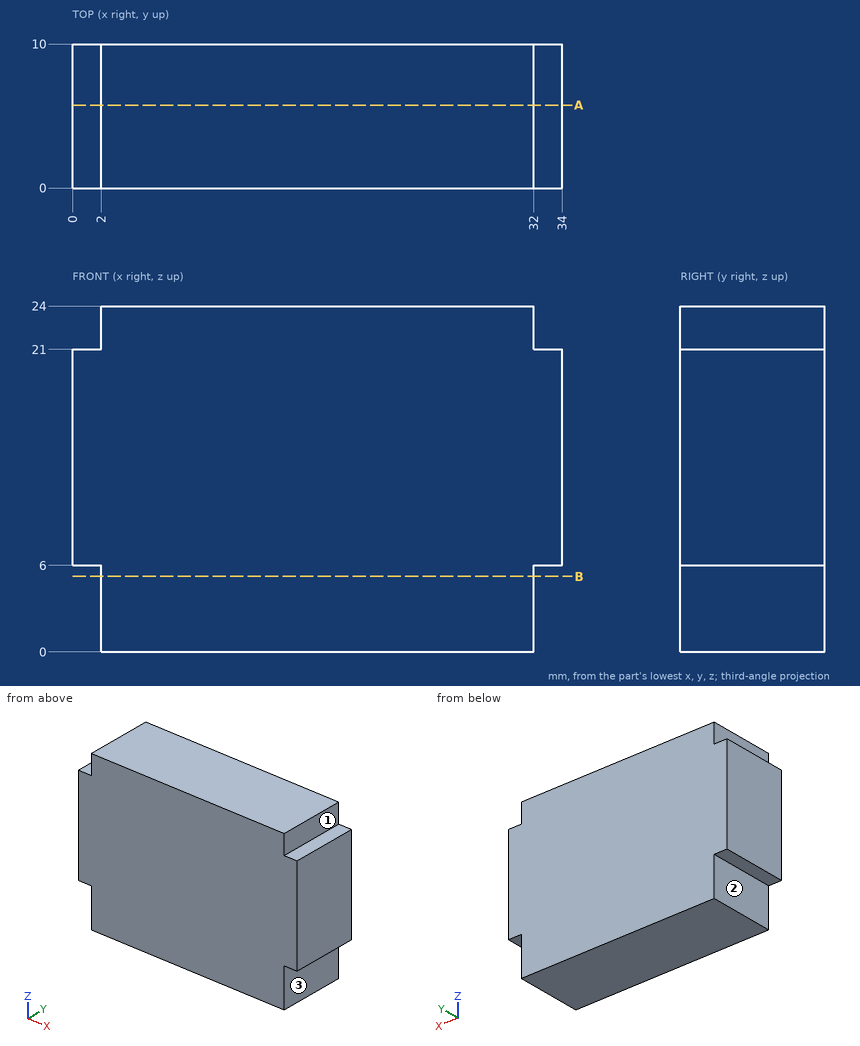
Here's the drawing with two shaded views (mm, measured from the low corner). I have some questions. A direction names the side the tool comes from. Coordinates: 2 decimals unless noted, no trailing zeros. Loops run counter-clockwise (first coordinate to the right, second up) from the corner with the lowest first, then second, coordinate; pieces in that order, holes last. Notation, with made-up numbers: M 65,42 L 81,42 A27 cw 81,58 Z; hole C 67,87.5 d5. An arc over 180 degrees is marked long. Put each result on its own line as item: value. Start each with the question number.
(1) Which directions (+Z, -Z, +X, -X, +Y, -Y) give clear straight access to the entire face, cutting with the end or side of a thin tool? Please do the marked faces 1, 2 and 3.
(2) Imagine slicing it at A-A on y = 5.75. List the corners of the cut face in (x, z) for me, and give its area (3 significant figures).
(3) Imagine slicing it at B-B on z = 5.25. List the corners of the cut face in (x, y) for me.
(4) Will these pins go through, and if not, where does the flat tip stop? pin 1 Ø0.6 at (x, y) = (1, 3.5) entering from +Z; pin 2 Ø2 at (x, y) = (33.5, 5.5) entering from -Z; pin 3 Ø0.9 at (y, z) = (3.5, 23) entering from +X.
(5) I need wall thicknesses on probe 1 along X at (y, z) = (1.5, 2.75). Which ranges of the line are inside material? Lowest first, please.
Worked answers:
1. face 1: +Z, +X, +Y, -Y
1. face 2: -Z, -X, +Y, -Y
1. face 3: -Z, +X, +Y, -Y
2. outline: M 0,6 L 2,6 L 2,0 L 32,0 L 32,6 L 34,6 L 34,21 L 32,21 L 32,24 L 2,24 L 2,21 L 0,21 Z
2. area: 780 mm2
3. outline: M 2,0 L 32,0 L 32,10 L 2,10 Z
4. pin 1: stops at z = 21
4. pin 2: stops at z = 6
4. pin 3: stops at x = 32
5. probe 1: x = 2 to 32
